```python
from build123d import *

# Parameters (mm, degrees)
SKETCH1_W           = 72
SKETCH1_H           = 45
BOSS_EXTRUDE1_DEPTH = 25
SKETCH2_R           = 5
CUT_EXTRUDE1_DEPTH  = 50.267129001
SKETCH3_R           = 3
CUT_EXTRUDE2_DEPTH  = 50.267129001
SKETCH4_R           = 15
CUT_EXTRUDE3_DEPTH  = 12


with BuildPart() as part:
    # Sketch1 → Boss-Extrude1 (new body)
    with BuildSketch(Plane(origin=(0, 0, 0), x_dir=(1, 0, 0), z_dir=(0, 1, 0))):
        Rectangle(SKETCH1_W, SKETCH1_H)
    extrude(amount=BOSS_EXTRUDE1_DEPTH)

    # Sketch2 → Cut-Extrude1 (cut, through all)
    with BuildSketch(Plane(origin=(0, 25, 0), x_dir=(1, 0, 0), z_dir=(0, 1, 0))):
        with Locations(Location((0, 0, 0), (0, 0, 270))):
            Circle(SKETCH2_R)
    extrude(amount=-CUT_EXTRUDE1_DEPTH, mode=Mode.SUBTRACT)

    # Sketch3 → Cut-Extrude2 (cut, through all)
    with BuildSketch(Plane(origin=(0, 25, 0), x_dir=(1, 0, 0), z_dir=(0, 1, 0))):
        with Locations(Location((-26, 0, 0), (0, 0, 270))):
            Circle(SKETCH3_R)
        with Locations(Location((26, 0, 0), (0, 0, 90))):
            Circle(SKETCH3_R)
    extrude(amount=-CUT_EXTRUDE2_DEPTH, mode=Mode.SUBTRACT)

    # Sketch4 → Cut-Extrude3 (cut)
    with BuildSketch(Plane(origin=(0, 25, 0), x_dir=(1, 0, 0), z_dir=(0, 1, 0))):
        with Locations(Location((0, 0, 0), (0, 0, 270))):
            Circle(SKETCH4_R)
    extrude(amount=-CUT_EXTRUDE3_DEPTH, mode=Mode.SUBTRACT)


solid = part.part
```
Input: part model. Units: mm. Frame: model coordinates. A direction names the side the tool comes from. Round coordinates to 2 decimals unless told otherwise and drop trailing zeros. Write each loop counter-clockwise with the first axis right and the second up, starting at its lowest first coordinate (ties: lowest second). Pieces come first, ordered by that corner, then holes. Notation, with made-up numbers: (-7.75, 82) - (-3.75, 82) arc R31 cw to (-3.75, 119) - close; hole circle Ø2 at (-37.75, 20.25). An arc over 180 degrees is marked (long way). Write item = value, one per line.
(1) Access query for faces 1 (the cylindrical face through (0.66, 19.084, -14.985)), 2 (the cylindrical face through (-4.88, 6.59, -1.08)). Directions: +Z, -Z, +X, -X, +Y, -Y. A direction counts if a zero-diameter tool reaches every point of the face in a straight line with its end or side. Return the directions, or none.
Geometry check:
face_1 = +Y
face_2 = +Y, -Y
(2) Section query D-D on z = 10.5. Output: boundary loops of the cut face in (x, y).
Geometry check:
outline = (-36, 0) - (36, 0) - (36, 25) - (10.71, 25) - (10.71, 13) - (-10.71, 13) - (-10.71, 25) - (-36, 25) - close
(3) Section query B-B on y = 4. Output: boundary loops of the cut face in (x, z).
Geometry check:
outline = (-36, -22.5) - (36, -22.5) - (36, 22.5) - (-36, 22.5) - close; hole circle Ø6 at (-26, 0); hole circle Ø10 at (0, 0); hole circle Ø6 at (26, 0)
(4) Section query A-A on z = 0. Output: boundary loops of the cut face in (x, y).
Geometry check:
outline = (-36, 0) - (-29, 0) - (-29, 25) - (-36, 25) - close; (-23, 0) - (-5, 0) - (-5, 13) - (-15, 13) - (-15, 25) - (-23, 25) - close; (5, 0) - (23, 0) - (23, 25) - (15, 25) - (15, 13) - (5, 13) - close; (29, 0) - (36, 0) - (36, 25) - (29, 25) - close
(5) Material intervals for probe 1 along X at (y, z) = (6.5, 0); probe 2 along X at (y, z) = (16.25, 0); probe 3 along Z at (x, y) = (26, 13.5), sorted ascending.
Geometry check:
probe_1 = -36 to -29, -23 to -5, 5 to 23, 29 to 36
probe_2 = -36 to -29, -23 to -15, 15 to 23, 29 to 36
probe_3 = -22.5 to -3, 3 to 22.5
(6) Pull-direction query (Z, two-part tool) for faces 3 (the flat face through (-36, 12, 0)), 4 (the flat face through (-1, 12, 22.5)), 5 (the flat face through (4, 13, -4)); classes: +Z half, -Z half, draft (parallel to the pull), parting line (faces both ways), or undercut.
Geometry check:
face_3 = draft
face_4 = +Z half
face_5 = undercut
(7) Section query C-C on x = 0. Output: boundary loops of the cut face in (y, z), then the cut area to 3 significant figures.
Geometry check:
outline = (0, -22.5) - (25, -22.5) - (25, -15) - (13, -15) - (13, -5) - (0, -5) - close; (0, 5) - (13, 5) - (13, 15) - (25, 15) - (25, 22.5) - (0, 22.5) - close
area = 635 mm^2
(8) Contact query for flat-ended pins moving along their axis: pin 1 Ø8 at (x, z) = (-1.5, -5.5) entering from -Y; pin 2 Ø15 at (x, z) = (-5.5, 4.5) entering from +Y. Output: stop coordinate, or through.
Geometry check:
pin_1 = 0
pin_2 = 13
